from build123d import *

# Parameters (mm, degrees)
SKETCH1_R                          = 20
EXTRUDE1_DEPTH                     = 12.0142
CHAMFER1_SIZE                      = 1.52
F_3_16_0_1875_DIAMETER_HOLE1_D     = 4.7625
F_3_16_0_1875_DIAMETER_HOLE1_DEPTH = 6.2484
SKETCH5_R                          = 18.984
EXTRUDE2_DEPTH                     = 0.98552
M5X0_8_TAPPED_HOLE1_D              = 4.2
M5X0_8_TAPPED_HOLE1_DEPTH          = 12.7
M5X0_8_TAPPED_HOLE1_TIP            = 1.2618073
CIRPATTERN1_COUNT                  = 3
SKETCH10_R                         = 3.937
CUT_EXTRUDE3_DEPTH                 = 0.381


with BuildPart() as part:
    # Sketch1 → Extrude1 (new body)
    with BuildSketch(Plane(origin=(0, 0, 0), x_dir=(1, 0, 0), z_dir=(0, 1, 0))):
        with Locations(Location((0, 0, 0), (0, 0, 270))):  # turned: the seam where the file's is
            Circle(SKETCH1_R)
    extrude(amount=EXTRUDE1_DEPTH)

    # Chamfer1
    chamfer1_edges = [part.edges().sort_by_distance(p)[0] for p in [
        (0, 12.0142, -20),
    ]]
    chamfer(chamfer1_edges, length=CHAMFER1_SIZE)

    # Sketch2 → Cut-Revolve1 (revolve, cut)
    with BuildSketch(Plane.XY):
        with BuildLine():
            Line((0, 19.0246), (0, 6.0198))
            ThreePointArc((0, 6.0198), (-6.5024, 12.5222), (0, 19.0246))
        make_face()
    revolve(axis=Axis((0, 19.0246, 0), (0, -1, 0)), mode=Mode.SUBTRACT)

    # 3_16 _0.1875_ Diameter Hole1
    with Locations(Plane(origin=(0, 12.0142, 0), x_dir=(-1, 0, 0), z_dir=(0, 1, 0))):
        with Locations((0, 0)):
            Hole(F_3_16_0_1875_DIAMETER_HOLE1_D / 2, depth=F_3_16_0_1875_DIAMETER_HOLE1_DEPTH)

    # Sketch5 → Extrude2 (add)
    with BuildSketch(Plane.XZ):
        with Locations(Location((0, 0, 0), (0, 0, 90))):  # turned: the seam where the file's is
            Circle(SKETCH5_R)
    extrude(amount=EXTRUDE2_DEPTH)

    # M5x0.8 Tapped Hole1
    with Locations(Plane(origin=(20, 6.6802, 0), x_dir=(0, 0, 1), z_dir=(1, 0, 0))):
        with Locations((0, 0)):
            Hole(M5X0_8_TAPPED_HOLE1_D / 2, depth=M5X0_8_TAPPED_HOLE1_DEPTH)
            with Locations((0, 0, -(M5X0_8_TAPPED_HOLE1_DEPTH + M5X0_8_TAPPED_HOLE1_TIP / 2))):  # 118° drill point
                Cone(0, M5X0_8_TAPPED_HOLE1_D / 2, M5X0_8_TAPPED_HOLE1_TIP, mode=Mode.SUBTRACT)

    # Sketch8 → M3x0.5 Tapped Hole1 (revolve, cut)
    with BuildSketch(Plane(origin=(-10.795, 12.0142, 0), x_dir=(0, 0, 1), z_dir=(1, 0, 0))):
        Polygon((0, 0), (0, 5.553072774), (1.25, 4.801997), (1.25, 3.302), (1.5, 3.302), (1.5, 0), align=None)
    m3x0_5_tapped_hole1 = revolve(axis=Axis((-10.795, 18.3642, 0), (0, -1, 0)), mode=Mode.SUBTRACT)

    # CirPattern1: M3x0.5 Tapped Hole1 ×3 about axis
    cirpattern1_axis = Axis((0, 0, 0), (0, 1, 0))
    for i in range(1, CIRPATTERN1_COUNT):
        add(m3x0_5_tapped_hole1.rotate(cirpattern1_axis, i * 360 / CIRPATTERN1_COUNT), mode=Mode.SUBTRACT)

    # Sketch10 → Cut-Extrude3 (cut)
    with BuildSketch(Plane(origin=(20, 5.2471, 0), x_dir=(0, 0, 1), z_dir=(1, 0, 0))):
        with Locations((0, -1.4331)):
            Circle(SKETCH10_R)
    extrude(amount=-CUT_EXTRUDE3_DEPTH, mode=Mode.SUBTRACT)


solid = part.part
Verification items for the finished model (mm, model axes). A direction names the side the tool comes from. Give positions to 0.01 mm unless a question says otherwise; leave off trailing zeros. Write each loop counter-clockwise with the first axis right and the second up, starting at its lowest first coordinate (ties: lowest second). Pieces come first, ordered by that corner, then holes.
(1) Access from +Z, -Z, +X, -X, +Y, -Y to the whole of each face (thin tool, end or side, straight path). Record for faces 1 (the face through (19.619, 8, 2)), 2 (the face through (4.55, 7.97, -10.27)), 3 (the face through (-19.524, 5.174, -4.336)).
(2) Material ranges on line 1 (X direction, y = 8.35, z = 0) (1 decimal); line 2 (X direction, y = 8.2, z = 0) (3 decimals); line 3 (Y direction, x = 11, z = 0), recorded low to high.
(3) Cross-section at B-B (y = 0.5). Enter the section's corners in (x, z).
(4) Mould release check, pull along Y, two halves, no side actions. Record for faces 4 (the face through (-1.89, 6.11, -1.45)), 5 (the face through (-10.71, 6.59, 0.2)), 6 (the face through (6.26, 7.04, -0.08)): +Y half, -Y half, draft (parallel to the pull), parting line (faces both ways), or undercut.
(5) Cross-section at C-C (y = 3.5). Enter the section's corners in (x, z).
(6) Cross-section at A-A (x = 0). Enter the section's corners in (y, z).
(7) Gauge pin test, flat ends, axial feed: pin 1 (4 mm diameter, centred on y = 1, z = -10.5, fed in from +X); pin 2 (6 mm diameter, centred on x = 5, y = 6.5, fed in from -Z); pin 3 (2 mm diameter, centred on x = 5.4, z = -9.35, fed in from +Y). Record the tip position at first contact, or that the pin passes through.
Worked out:
1. face 1: +X
1. face 2: +Y
1. face 3: +Y, -Y
2. line 1: x = -20 to -12, -9.5 to -5, 5 to 7
2. line 2: x = -20 to -12.045, -9.545 to -4.858, 4.858 to 6.951
2. line 3: y = -0.99 to 4.58, 8.78 to 12.01
3. outline: circle Ø40 at (0, 0)
4. face 4: draft
4. face 5: +Y half
4. face 6: undercut
5. outline: (19.62, -2.32) - (19.62, 2.32) - (19.86, 2.32) arc R20 ccw (long way) to (19.86, -2.32) - close
6. outline: (-0.99, -18.98) - (0, -18.98) - (0, -20) - (10.49, -20) - (12.01, -18.48) - (12.01, -6.48) arc R6.5 cw to (6.47, -2.38) - (5.77, -2.38) - (5.77, 2.38) - (6.47, 2.38) arc R6.5 cw to (12.01, 6.48) - (12.01, 18.48) - (10.49, 20) - (0, 20) - (0, 18.98) - (-0.99, 18.98) - close
7. pin 1: stops at x = 18.1
7. pin 2: stops at z = -19.9
7. pin 3: stops at y = 7.06
